Source: CAD feature listing. Evaluate the final solid. Frame: model axes, mm. Face numbers are marked on the shaded views. A direction names the side the tool comes from. Round coordinates to 2 decimals unless told otherwise and drop trailing zeros. Loops run counter-clockwise (first coordinate to the right, second up) from the corner with the lowest first, then second, coordinate; pieces in that order, holes last. Notation, with made-up numbers: (53, 76) -> (77, 76) arc R8 cw to (77, 81) -> close; hole circle Ø7 at (29.25, 5.25). An arc over 180 degrees is marked (long way). Put each result on its own line as item: value. Start each with the question number.
1. Contact query for flat-ended pins moving along their axis: pin 1 (0.8 mm diameter, centred on x = 7.5, z = -1, fed in from +Y); pin 2 (3 mm diameter, centred on x = 1, y = 26, fed in from +Z); pin 3 (1.2 mm diameter, centred on x = 1, y = 27.5, fed in from -Z); pin 4 (1 mm diameter, centred on x = -4, y = 21.5, fed in from +Z). Output: stop coordinate, or through.
2. Cut plane A-A (y = 14.25). Return the cut outline in (x, z).
3. Cut plane B-B (x = 0). Return the cut outline in (y, z), then the cut area to 3 significant figures.
4. Set-up query: the marked faces 1, 2, 3 and 4. Return all of +Z, -Z, +X, -X, +Y, -Y with unobstructed straight access to the full face (end or side cutting, diameter ignored); none if empty.
5. Material intervals for L1, parallel to Z at x = 0.25, y = 9.25; L2, parallel to Y at x = -6.5, z = 3; L3, parallel to X at y = 15.75, z = -3.5, sorted ascending.
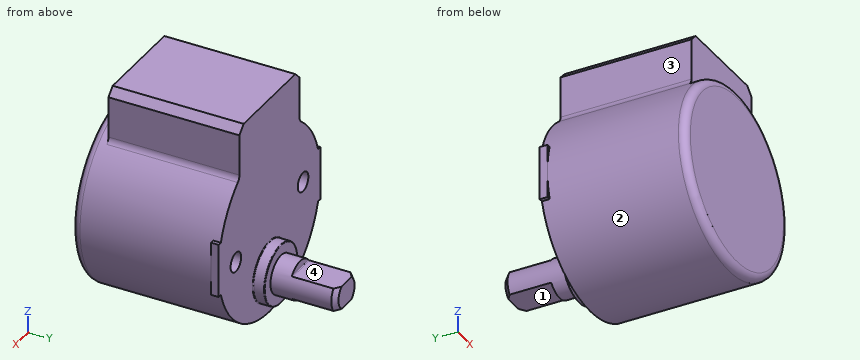
```python
from build123d import *

# Parameters (mm, degrees)
SKETCH1_R           = 12
BOSS_EXTRUDE1_DEPTH = 19
SKETCH2_W           = 14.2
SKETCH2_H           = 7.594673869
BOSS_EXTRUDE2_DEPTH = 17
SKETCH3_R           = 2.05
BOSS_EXTRUDE3_DEPTH = 1
CHAMFER1_SIZE       = 0.6
SKETCH5_W           = 6
SKETCH5_H           = 2
CUT_EXTRUDE1_DEPTH  = 6
FILLET1_R           = 0.1
CHAMFER2_SIZE       = 1
FILLET2_R           = 1
FILLET3_R           = 0.1
FILLET4_R           = 1
SKETCH6_W           = 9.256543548
SKETCH6_H           = 10.153653495
CUT_EXTRUDE2_DEPTH  = 32.531730051
SKETCH8_R           = 1.25
CUT_EXTRUDE3_DEPTH  = 3


with BuildPart() as part:
    # Sketch1 → Boss-Extrude1 (new body)
    with BuildSketch(Plane(origin=(0, 0, 0), x_dir=(1, 0, 0), z_dir=(0, 1, 0))):
        with Locations(Location((0, 0, 0), (0, 0, 270))):
            Circle(SKETCH1_R)
    extrude(amount=BOSS_EXTRUDE1_DEPTH)

    # Sketch2 → Boss-Extrude2 (add)
    with BuildSketch(Plane(origin=(0, 2, 0), x_dir=(-1, 0, 0), z_dir=(0, -1, 0))):
        with Locations((0, -12.702663066)):
            Rectangle(SKETCH2_W, SKETCH2_H)
    extrude(amount=-BOSS_EXTRUDE2_DEPTH)

    # Sketch3 → Boss-Extrude3 (add)
    # profile 1 of 2: a face of its own
    with BuildSketch(Plane(origin=(0, 19, 0), x_dir=(1, 0, 0), z_dir=(0, 1, 0))):
        with BuildLine():
            Line((-15.5, -3.5), (-8, -3.5))
            Line((-8, -3.5), (-8, 3.5))
            Line((-8, 3.5), (-15.5, 3.5))
            ThreePointArc((-15.5, 3.5), (-19, 0), (-15.5, -3.5))
        make_face()
        with Locations(Location((-15.5, 0, 0), (0, 0, 270))):
            Circle(SKETCH3_R, mode=Mode.SUBTRACT)
    # profile 2 of 2: a face of its own
    with BuildSketch(Plane(origin=(0, 19, 0), x_dir=(1, 0, 0), z_dir=(0, 1, 0))):
        with BuildLine():
            Line((8, -3.5), (8, 3.5))
            Line((8, 3.5), (15.5, 3.5))
            ThreePointArc((15.5, 3.5), (19, 0), (15.5, -3.5))
            Line((15.5, -3.5), (8, -3.5))
        make_face()
        with Locations(Location((15.5, 0, 0), (0, 0, 90))):
            Circle(SKETCH3_R, mode=Mode.SUBTRACT)
    extrude(amount=-BOSS_EXTRUDE3_DEPTH)

    # Sketch4 → Revolve1 (revolve)
    with BuildSketch(Plane(origin=(0, 0, 0), x_dir=(0, 0, -1), z_dir=(1, 0, 0))):
        Polygon((6.5, 19), (2.6, 19), (2.6, 20.5), (4, 20.5), (4, 29), (6.5, 29), align=None)
    revolve(axis=Axis((0, 23.531707116, -6.5), (0, -1, 0)))

    # Chamfer1
    chamfer1_edges = [part.edges().sort_by_distance(p)[0] for p in [
        (0, 29, -9),
    ]]
    chamfer(chamfer1_edges, length=CHAMFER1_SIZE)

    # Sketch5 → Cut-Extrude1 (cut)
    with BuildSketch(Plane(origin=(0, 29, 0), x_dir=(1, 0, 0), z_dir=(0, 1, 0))):
        with Locations((0, 9)):
            Rectangle(SKETCH5_W, SKETCH5_H)
        with Locations((0, 4)):
            Rectangle(SKETCH5_W, SKETCH5_H)
    extrude(amount=-CUT_EXTRUDE1_DEPTH, mode=Mode.SUBTRACT)

    # Fillet1
    fillet1_edges = [part.edges().sort_by_distance(p)[0] for p in [
        (0, 23, -8),
        (0, 23, -5),
    ]]
    fillet(fillet1_edges, radius=FILLET1_R)

    # Chamfer2
    chamfer2_edges = [part.edges().sort_by_distance(p)[0] for p in [
        (-7.1, 10.5, 16.5),
        (7.1, 10.5, 16.5),
    ]]
    chamfer(chamfer2_edges, length=CHAMFER2_SIZE)

    # Fillet2
    fillet2_edges = [part.edges().sort_by_distance(p)[0] for p in [
        (7.1, 10.5, 9.674192473),
        (-7.1, 10.5, 9.674192473),
    ]]
    fillet(fillet2_edges, radius=FILLET2_R)

    # Fillet3
    fillet3_edges = [part.edges().sort_by_distance(p)[0] for p in [
        (0, 19, -10.4),
        (0, 20.5, -10.4),
    ]]
    fillet(fillet3_edges, radius=FILLET3_R)

    # Fillet4
    fillet4_edges = [part.edges().sort_by_distance(p)[0] for p in [
        (0, 0, -12),
    ]]
    fillet(fillet4_edges, radius=FILLET4_R)

    # Sketch6 → Cut-Extrude2 (cut, through all)
    with BuildSketch(Plane(origin=(0, 19, 0), x_dir=(1, 0, 0), z_dir=(0, 1, 0))):
        with Locations((-16.628271774, -0.333446931)):
            Rectangle(SKETCH6_W, SKETCH6_H)
        with Locations((16.628271774, -0.333446931)):
            Rectangle(SKETCH6_W, SKETCH6_H)
    extrude(amount=-CUT_EXTRUDE2_DEPTH, mode=Mode.SUBTRACT)

    # Sketch8 → Cut-Extrude3 (cut)
    with BuildSketch(Plane(origin=(0, 19, 0), x_dir=(1, 0, 0), z_dir=(0, 1, 0))):
        with Locations(Location((-7.931558639, -1.044209433, 0), (0, 0, 270))):
            Circle(SKETCH8_R)
        with Locations(Location((7.931559171, 1.044209433, 0), (0, 0, 270))):
            Circle(SKETCH8_R)
    extrude(amount=-CUT_EXTRUDE3_DEPTH, mode=Mode.SUBTRACT)


solid = part.part
```
Solution:
1. pin 1: stops at y = 16
1. pin 2: stops at z = -5
1. pin 3: stops at z = -8
1. pin 4: passes through
2. outline: (-7.48, 9.39) arc R12 ccw (long way) to (7.48, 9.39) arc R1 cw to (7.1, 10.17) -> (7.1, 15.5) -> (6.1, 16.5) -> (-6.1, 16.5) -> (-7.1, 15.5) -> (-7.1, 10.17) arc R1 cw to start
3. outline: (0, -11) arc R1 ccw to (1, -12) -> (19, -12) -> (19, -10.5) arc R0.1 cw to (19.1, -10.4) -> (20.4, -10.4) arc R0.1 ccw to (20.5, -10.3) -> (20.5, -9) -> (23, -9) -> (23, -8.1) arc R0.1 cw to (23.1, -8) -> (29, -8) -> (29, -5) -> (23.1, -5) arc R0.1 cw to (23, -4.9) -> (23, -4) -> (20.5, -4) -> (20.5, -2.7) arc R0.1 ccw to (20.4, -2.6) -> (19.1, -2.6) arc R0.1 cw to (19, -2.5) -> (19, 16.5) -> (2, 16.5) -> (2, 12) -> (1, 12) arc R1 ccw to (0, 11) -> close
3. area: 574 mm^2
4. face 1: -Z, +X, -X, +Y
4. face 2: -Y
4. face 3: +Z, -X, +Y, -Y
4. face 4: +Z, +X, -X, +Y
5. L1: z = -12 to 16.5
5. L2: y = 0 to 19
5. L3: x = -11.48 to 11.48
